Autodesk Inventor part; units mm, degrees
ref_plane "YZ Plane" through (0, 0, 0) normal (1, 0, 0) x (0, 1, 0)
ref_plane "XZ Plane" through (0, 0, 0) normal (0, 1, 0) x (-1, 0, 0)
ref_plane "XY Plane" through (0, 0, 0) normal (0, 0, 1) x (1, 0, 0)
sketch "Skizze1" plane through (0, 0, 0) normal (0, 0, 1) x (1, 0, 0)
  line L0 (0, 0) -> (0, 61)
  line L1 (25, 0) -> (25, 61)
  line L2 (0, 61) -> (-5, 61)
  line L3 (25, 61) -> (30, 61)
  line L4 (-5, 61) -> (-5, 0)
  line L5 (-5, 0) -> (0, 0)
  line L6 (30, 61) -> (30, 0)
  line L7 (30, 0) -> (25, 0)
  dimension "d1" = 61
  dimension "d2" = 61
  dimension "d3" = 25
  dimension "d4" = 5
  dimension "d5" = 5
extrude "Extrusion1" add sketch "Skizze1" along normal blind 55
sketch "Skizze2" plane through (0, 0, 0) normal (1, 0, 0) x (0, 0, -1)
  line L0 (-55, 61) -> (-55, 0)
  line L1 (0, 0) -> (-55, 0)
  line L2 (-55, 61) -> (-53, 61)
  line L3 (-53, 61) -> (-53, 0)
  line L4 (-53, 0) -> (-55, 0)
  line L5 (-55, 0) -> (-55, 61)
  dimension "d8" = 2
extrude "Extrusion2" add sketch "Skizze2" along normal blind 25
sketch "Skizze3" plane through (0, 0, 55) normal (0, 0, 1) x (1, 0, 0)
  circle A0 centre (12.5, 30.5) radius 5.5
  line L0 (30, 61) -> (-5, 61)
  line L1 (30, 0) -> (30, 61)
  line L2 (30, 0) -> (-5, 0)
  line L3 (-5, 0) -> (-5, 61)
  line L4 (30, 61) -> (-5, 61)
  line L5 (-5, 61) -> (-5, 0)
  line L6 (-5, 0) -> (30, 0)
  line L7 (30, 0) -> (30, 61)
  line L8 (30, 61) -> (30, 0)
  line L9 (-5, 61) -> (30, 61)
  point P0 (0, 0)
  dimension "d11" = 30.5
  dimension "d12" = 17.5
  dimension "d13" = 11
extrude "Extrusion3" cut sketch "Skizze3" against normal blind 2.5 contours A0
sketch "Skizze4" plane through (0, 0, 55) normal (0, 0, 1) x (1, 0, 0)
  circle A0 centre (12.5, 30.5) radius 5.5
  circle A1 centre (12.5, 30.5) radius 5.5
  circle A2 centre (12.5, 30.5) radius 5.5
  line L0 (-9.5, 27) -> (-9.5, 20)
  line L1 (34.5, 27) -> (34.5, 20)
  line L2 (30, 61) -> (30, 0)
  line L3 (-5, 61) -> (-5, 0)
  line L4 (-9.5, 27) -> (-2.5, 27)
  line L5 (27.5, 27) -> (34.5, 27)
  line L6 (-9.5, 20) -> (-2.5, 20)
  line L7 (27.5, 20) -> (34.5, 20)
  line L8 (-2.5, 20) -> (-2.5, 27)
  line L9 (27.5, 27) -> (27.5, 20)
  line L10 (30, 61) -> (30, 0)
  line L11 (30, 0) -> (-5, 0)
  line L12 (-5, 0) -> (-5, 61)
  line L13 (-5, 61) -> (30, 61)
  line L14 (30, 61) -> (30, 0)
  line L15 (30, 0) -> (-5, 0)
  line L16 (-5, 0) -> (-5, 61)
  line L17 (-5, 61) -> (30, 61)
  line L18 (30, 61) -> (30, 0)
  line L19 (30, 0) -> (-5, 0)
  line L20 (-5, 0) -> (-5, 61)
  line L21 (-5, 61) -> (30, 61)
  point P0 (0, 0)
  point P1 (27.5, 61)
  point P2 (27.5, 0)
  point P3 (-2.5, 0)
  point P4 (-2.5, 61)
  dimension "d29" = 7
  dimension "d30" = 7
  dimension "d31" = 7
  dimension "d32" = 7
extrude "Extrusion4" add sketch "Skizze4" against normal blind 20 contours L4 L3 L6 L0 | L4 L8 L6 L3 | L5 L1 L7 L2 | L2 L7 L9 L5
sketch "Skizze5" plane through (0, 0, 55) normal (0, 0, 1) x (1, 0, 0)
  circle A0 centre (-5, 23.5) radius 1.9403
  circle A1 centre (30, 23.5) radius 2.0247
  circle A2 centre (12.5, 30.5) radius 5.5
  line L0 (-9.5, 20) -> (-9.5, 27)
  dimension "d25" = 35
  dimension "d27" = 7
  dimension "d28" = 7
  dimension "d33" = 17.5
extrude "Extrusion5" cut sketch "Skizze5" against normal blind 15 contours A0 | A1
sketch "Skizze6" plane through (30, 0, 0) normal (1, 0, 0) x (0, 0, -1)
  line L0 (-17.5, 40.25) -> (-11.5, 40.25)
  line L1 (-11.5, 40.25) -> (-11.5, 20.75)
  line L2 (-11.5, 20.75) -> (-17.5, 20.75)
  line L3 (-17.5, 20.75) -> (-17.5, 40.25)
  line L4 (0, 61) -> (0, 0)
  line L5 (0, 0) -> (-55, 0)
  line L6 (-55, 27) -> (-35, 27)
  line L7 (-35, 27) -> (-35, 20)
  line L8 (-35, 20) -> (-55, 20)
  line L9 (-55, 0) -> (-55, 20)
  line L10 (0, 0) -> (-55, 0)
  line L11 (0, 61) -> (0, 0)
  line L12 (0, 61) -> (-55, 61)
  line L13 (-55, 27) -> (-55, 61)
  point P0 (-17.5, 30.5)
  dimension "d36" = 6
  dimension "d37" = 19.5
  dimension "d38" = 11.5
  dimension "d40" = 30.5
extrude "Extrusion6" cut sketch "Skizze6" against normal blind 35 contours L0 L1 L2 L3
sketch "Skizze8" plane through (0, 0, 0) normal (0, 0, -1) x (-1, 0, 0)
  line L0 (0, 20.75) -> (0, 40.25)
  line L1 (1, 35.5) -> (0, 35.5)
  line L2 (0, 35.5) -> (0, 25.5)
  line L3 (0, 25.5) -> (1, 25.5)
  line L4 (1, 25.5) -> (1, 35.5)
  line L5 (0, 61) -> (5, 61)
  line L6 (-25, 0) -> (-25, 61)
  line L7 (-25, 35.5) -> (-26, 35.5)
  line L8 (-26, 35.5) -> (-26, 25.5)
  line L9 (-26, 25.5) -> (-25, 25.5)
  line L10 (-25, 25.5) -> (-25, 35.5)
  point P0 (0, 0)
  point P1 (1, 30.5)
  point P2 (13.2784, 51.1394)
  dimension "d43" = 1
  dimension "d44" = 10
  dimension "d45" = 30.5
  dimension "d46" = 1
extrude "Extrusion7" cut sketch "Skizze8" against normal blind 5
sketch "Skizze11" plane through (25, 0, 53) normal (-1, 0, 0) x (0, 0, 1)
  circle A0 centre (-43, 10) radius 3.5
  circle A1 centre (-43, 51) radius 3.5
  line L0 (-53, 61) -> (-53, 0)
  line L1 (-53, 0) -> (2, 0)
  line L2 (-53, 61) -> (2, 61)
  dimension "d63" = 7
  dimension "d64" = 7
  dimension "d65" = 10
  dimension "d66" = 10
  dimension "d67" = 10
  dimension "d68" = 10
sketch "Skizze12" plane through (0, 0, 53) normal (1, 0, 0) x (0, 0, -1)
  circle A0 centre (43, 10) radius 3.5
  circle A1 centre (43, 51) radius 3.5
  line L0 (53, 61) -> (53, 0)
  line L1 (53, 0) -> (-2, 0)
  line L2 (53, 61) -> (-2, 61)
  dimension "d69" = 7
  dimension "d70" = 7
  dimension "d71" = 10
  dimension "d72" = 10
  dimension "d73" = 10
  dimension "d74" = 10
extrude "Extrusion8" cut sketch "Skizze11" against normal blind 2
extrude "Extrusion9" cut sketch "Skizze12" against normal blind 2
properties part number "motor_mount"
The listing builds one solid part. Answer for the finished solid, in the listing's coordinates (mm). A direction names the side the tool comes from. Give positions to 0.01 mm unless a question says otherwise; leave off trailing zeros. Write each loop counter-clockwise with the first axis right and the second up, starting at its lowest first coordinate (ties: lowest second). Pieces come first, ordered by that corner, then holes. Notation, with made-up numbers: (36, -24) -> (75, -24) arc R5 ccw to (75, -15) -> close; hole circle Ø1 at (9, 40). An arc over 180 degrees is marked (long way). Use a Markdown table: item, result.
(1) Section D-D, the plane y = 30.5 is taken. Determine the outline of the cut face in (x, z).
Return value:
| item | result |
|---|---|
| outline | (-5, 0) -> (-1, 0) -> (-1, 5) -> (0, 5) -> (0, 11.5) -> (-5, 11.5) -> close; (-5, 17.5) -> (0, 17.5) -> (0, 53) -> (7, 53) -> (7, 55) -> (-5, 55) -> close; (18, 53) -> (25, 53) -> (25, 17.5) -> (30, 17.5) -> (30, 55) -> (18, 55) -> close; (25, 5) -> (26, 5) -> (26, 0) -> (30, 0) -> (30, 11.5) -> (25, 11.5) -> close |
(2) Find the intervals of material crossed by probe 1 along Y at (x, z) = (-0.6, 10); probe 2 along X at (y, z) = (37.5, 24.5); probe 3 along Z at (x, y) = (-3.5, 27), in increasing order. Write a range as from..to.
Return value:
| item | result |
|---|---|
| probe 1 | 0..6.5, 13.5..47.5, 54.5..61 |
| probe 2 | -5..0, 25..30 |
| probe 3 | 0..11.5, 17.5..55 |
(3) Determine the mould class of faces 6 (the flat face through (34.5, 24, 45)), 7 (the flat face through (32, 24, 35)), 8 (the cylindrical face through (-0.986, 6.583, 10.759)) for opening direction Z: released by +Z, released by -Z, zero draft, split by the parting line, or undercut.
Return value:
| item | result |
|---|---|
| face 6 | zero draft |
| face 7 | released by -Z |
| face 8 | undercut |
(4) For faces 1 (the flat face through (-1, 30, 2)), 2 (the flat face through (28, 30, 17.5)), 3 (the flat face through (32, 20, 45)), 4 (the cylindrical face through (26, 7.9, 7.2)), 5 (the flat face through (25, 30, 26)), determine the directions among +Z, -Z, +X, -X, +Y, -Y from which every point of the face is accessible in a straight line to the end or side of a thin tool.
Return value:
| item | result |
|---|---|
| face 1 | -Z |
| face 2 | +X, -X |
| face 3 | +Z, -Z, +X, -Y |
| face 4 | none |
| face 5 | -Z, +Y, -Y |
(5) Flat-ended cylindrical pins translate along their axes: P1, Ø4, axis at x = 8, y = 28.5, coming from the -Z side; P2, Ø5.5, axis at y = 10, z = 10, coming from the +X side; P3, Ø7.5, axis at y = 9, z = 8.5, coming from the -X side; P4, Ø2.5, axis at x = 28.5, z = 16, coming from the -Y side. Find the tip coordinate at first contact, or state that the pin passes through.
Return value:
| item | result |
|---|---|
| P1 | z = 53 |
| P2 | x = 30 |
| P3 | x = -5 |
| P4 | y = 0 |
(6) Section A-A, the plane z = 48 is taken. Determine the outline of the cut face in (x, y).
Return value:
| item | result |
|---|---|
| outline | (-9.5, 20) -> (-5, 20) -> (-5, 0) -> (0, 0) -> (0, 61) -> (-5, 61) -> (-5, 27) -> (-9.5, 27) -> close; (25, 0) -> (30, 0) -> (30, 20) -> (34.5, 20) -> (34.5, 27) -> (30, 27) -> (30, 61) -> (25, 61) -> close; hole circle Ø3.88 at (-5, 23.5); hole circle Ø4.05 at (30, 23.5) |
(7) Section B-B, the plane x = 12.5 is taken. Determine the outline of the cut face in (y, z).
Return value:
| item | result |
|---|---|
| outline | (0, 53) -> (25, 53) -> (25, 55) -> (0, 55) -> close; (36, 53) -> (61, 53) -> (61, 55) -> (36, 55) -> close |
(8) Section C-C, the plane z = 10 is taken. Determine the outline of the cut face in (x, y).
Return value:
| item | result |
|---|---|
| outline | (-5, 0) -> (0, 0) -> (0, 6.5) -> (-2, 6.5) -> (-2, 13.5) -> (0, 13.5) -> (0, 47.5) -> (-2, 47.5) -> (-2, 54.5) -> (0, 54.5) -> (0, 61) -> (-5, 61) -> close; (25, 0) -> (30, 0) -> (30, 61) -> (25, 61) -> (25, 54.5) -> (27, 54.5) -> (27, 47.5) -> (25, 47.5) -> (25, 13.5) -> (27, 13.5) -> (27, 6.5) -> (25, 6.5) -> close |
